```python
from build123d import *

# Parameters (mm, degrees)
SKETCH2_W           = 17
SKETCH2_H           = 10
SKETCH2_R           = 1.5
SKETCH2_W_2         = 10
SKETCH2_H_2         = 22.35
BOSS_EXTRUDE1_DEPTH = 3
FILLET5_R           = 1
FILLET6_R           = 1
FILLET7_R           = 1


with BuildPart() as part:
    # Sketch2 → Boss-Extrude1 (new body)
    # profile 1 of 2: a face of its own
    with BuildSketch(Plane.XY):
        Rectangle(SKETCH2_W, SKETCH2_H)
        Circle(SKETCH2_R, mode=Mode.SUBTRACT)
    # profile 2 of 2: a face of its own
    with BuildSketch(Plane.XY):
        with Locations((0, -16.175)):
            Rectangle(SKETCH2_W_2, SKETCH2_H_2)
        with Locations((0, -7.3)):
            Circle(SKETCH2_R, mode=Mode.SUBTRACT)
        with Locations((0, -25.05)):
            Circle(SKETCH2_R, mode=Mode.SUBTRACT)
    extrude(amount=BOSS_EXTRUDE1_DEPTH)

    # Fillet5
    fillet5_edges = [part.edges().sort_by_distance(p)[0] for p in [
        (8.5, -5, 1.5),
    ]]
    fillet(fillet5_edges, radius=FILLET5_R)

    # Fillet6
    fillet6_edges = [part.edges().sort_by_distance(p)[0] for p in [
        (5, -27.35, 1.5),
        (-5, -27.35, 1.5),
        (-8.5, -5, 1.5),
    ]]
    fillet(fillet6_edges, radius=FILLET6_R)

    # Fillet7
    fillet7_edges = [part.edges().sort_by_distance(p)[0] for p in [
        (8.5, 5, 1.5),
        (-8.5, 5, 1.5),
    ]]
    fillet(fillet7_edges, radius=FILLET7_R)


solid = part.part
```
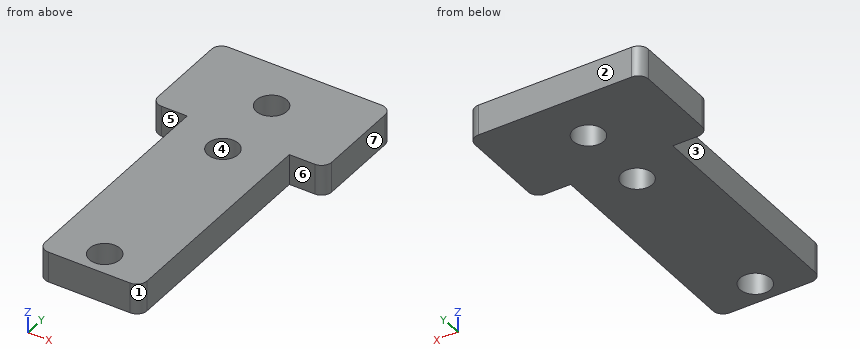
Part model, mm, in its own coordinate system. Face numbers are marked on the shaded views. A direction names the side the tool comes from. Round coordinates to 2 decimals unless told otherwise and drop trailing zeros. Write each loop counter-clockwise with the first axis right and the second up, starting at its lowest first coordinate (ties: lowest second). Pieces come first, ordered by that corner, then holes. Notation, with made-up numbers: (-25.5, 17.5) -> (-19.5, 17.5) arc R21 ccw to (-19.5, 31.5) -> close; hole circle Ø6 at (31.25, 14). An arc over 180 degrees is marked (long way). Return JSON: item names as keys, results as strings. Group by question number.
Q1. Which spindle directions (+Z, -Z, +X, -X, +Y, -Y) get a long thin tool onto all of the face, cutting with end or side? Do the marked faces 5, 6 and 7. Say none if no direction does.
Q2. Pin check, flat tips, straight feed: pin 1 (1 mm diameter, centred on x = 6, z = 2.5, fed in from -Y); pin 2 (2.5 mm diameter, centred on x = 0, y = -7.3, fed in from +Z). Stop position of each tip, or through.
Q3. Saw through at B-B on z = 1. Write the cut outline in (x, y).
Q4. Saw through at A-A on y = 0. Write the cut outline in (x, z), plus the area to 3 significant figures.
Q5. Mould opens along X. For the marked faces 1, 2, 3 and 4 say: pulls with the +X half, pulls with the -X half, needs draft (parallel to the pull), parting line crosses it, or undercut.
Q6. Probe L1, parallel to Y at x = 0, z = 0.95; L2, parallel to Y at x = -0.5, z = 0.3; L3, parallel to X at y = -25, z = 1.85. List the from-to ranges inside material, lowest first. Write a range as [from, to].
Q7. Saw through at D-D on y = -25.05. Write the cut outline in (x, z), plus the area to 3 significant figures.
Q8. Saw through at C-C on x = 0. Write the cut outline in (y, z), plus the area to 4 significant figures.
Answer:
{
 "1": {"face 5": "+Z, -Z, -X, -Y", "face 6": "+Z, -Z, +X, -Y", "face 7": "+Z, -Z, +X, +Y, -Y"},
 "2": {"pin 1": "y = -5", "pin 2": "through"},
 "3": {"outline": "(-8.5, -4) arc R1 ccw to (-7.5, -5) -> (-5, -5) -> (-5, -26.35) arc R1 ccw to (-4, -27.35) -> (4, -27.35) arc R1 ccw to (5, -26.35) -> (5, -5) -> (7.5, -5) arc R1 ccw to (8.5, -4) -> (8.5, 4) arc R1 ccw to (7.5, 5) -> (-7.5, 5) arc R1 ccw to (-8.5, 4) -> close; hole circle Ø3 at (0, -25.05); hole circle Ø3 at (0, -7.3); hole circle Ø3 at (0, 0)"},
 "4": {"outline": "(-8.5, 0) -> (-1.5, 0) -> (-1.5, 3) -> (-8.5, 3) -> close; (1.5, 0) -> (8.5, 0) -> (8.5, 3) -> (1.5, 3) -> close", "area": "42.0 mm2"},
 "5": {"face 1": "pulls with the +X half", "face 2": "needs draft", "face 3": "pulls with the -X half", "face 4": "undercut"},
 "6": {"L1": "[-27.35, -26.55], [-23.55, -8.8], [-5.8, -1.5], [1.5, 5]", "L2": "[-27.35, -26.46], [-23.64, -8.71], [-5.89, -1.41], [1.41, 5]", "L3": "[-5, -1.5], [1.5, 5]"},
 "7": {"outline": "(-5, 0) -> (-1.5, 0) -> (-1.5, 3) -> (-5, 3) -> close; (1.5, 0) -> (5, 0) -> (5, 3) -> (1.5, 3) -> close", "area": "21.0 mm2"},
 "8": {"outline": "(-27.35, 0) -> (-26.55, 0) -> (-26.55, 3) -> (-27.35, 3) -> close; (-23.55, 0) -> (-8.8, 0) -> (-8.8, 3) -> (-23.55, 3) -> close; (-5.8, 0) -> (-1.5, 0) -> (-1.5, 3) -> (-5.8, 3) -> close; (1.5, 0) -> (5, 0) -> (5, 3) -> (1.5, 3) -> close", "area": "70.05 mm2"}
}
